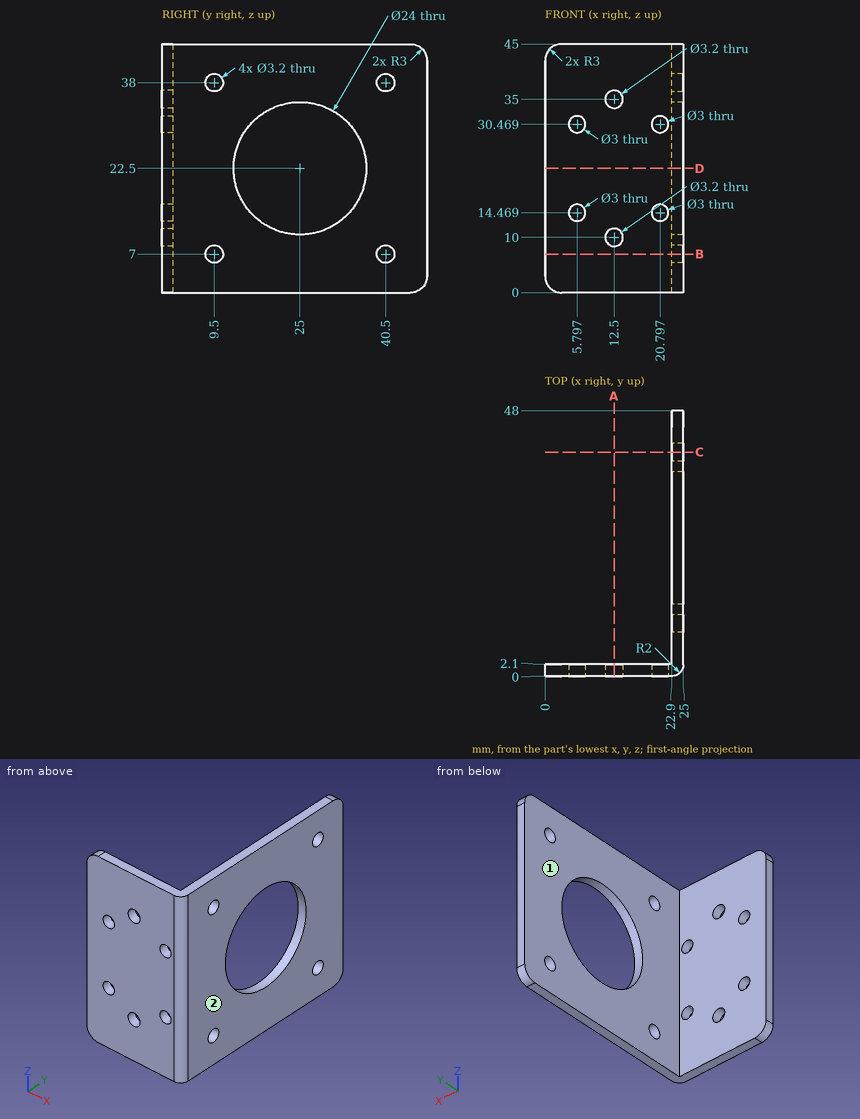
Part print with two shaded views. Sizes in mm from the minimum x, y, z corner. A direction names the side the tool comes from. Coordinates: 2 decimals unless noted, no trailing zeros. Write each loop counter-clockwise with the first axis right and the second up, starting at its lowest first coordinate (ties: lowest second). Pieces come first, ordered by that corner, then holes. Notation, with made-up numbers: M 34.5,28.25 L 45.5,28.25 A35 ccw 45.5,60.25 Z; hole C 66,-10 d5. An arc over 180 degrees is marked long. Return JSON: item names as keys, results as strings.
Item 1: Which spindle directions (+Z, -Z, +X, -X, +Y, -Y) get a long thin tool onto all of the face, cutting with end or side? Do the marked faces 1 and 2. Say none if no direction does.
Findings below:
{"face 1": "+Z, -Z, -X, +Y", "face 2": "+Z, -Z, +X, +Y, -Y"}
Item 2: Slice it at C-C, the plane y = 40.5. Write the cut outline in (x, z).
Findings below:
{"outline": "M 22.9,0 L 25,0 L 25,5.4 L 22.9,5.4 Z; M 22.9,8.6 L 25,8.6 L 25,36.4 L 22.9,36.4 Z; M 22.9,39.6 L 25,39.6 L 25,45 L 22.9,45 Z"}
Item 3: Slice it at D-D, the plane z = 22.5. Write the cut outline in (x, y).
Findings below:
{"outline": "M 0,0 L 23,0 A2 ccw 25,2 L 25,13 L 22.9,13 L 22.9,2.1 L 0,2.1 Z; M 22.9,37 L 25,37 L 25,48 L 22.9,48 Z"}
Item 4: Probe line 1 (Y direction, x = 12.5, z = 39); line 2 (X direction, y = 6, z = 30); line 3 (Y direction, x = 24.5, z = 22.5). List the from-to ranges inside material, lowest first. Write a range as from..to.
Findings below:
{"line 1": "y = 0..2.1", "line 2": "x = 22.9..25", "line 3": "y = 0.68..13, 37..48"}
Item 5: Slice it at B-B, the plane z = 7. Write the cut outline in (x, y), and give its area (3 significant figures).
Findings below:
{"outline": "M 0,0 L 23,0 A2 ccw 25,2 L 25,7.9 L 22.9,7.9 L 22.9,2.1 L 0,2.1 Z; M 22.9,11.1 L 25,11.1 L 25,38.9 L 22.9,38.9 Z; M 22.9,42.1 L 25,42.1 L 25,48 L 22.9,48 Z", "area": "135 mm2"}
Item 6: Slice it at A-A, the plane x = 12.5. Write the cut outline in (y, z).
Findings below:
{"outline": "M 0,0 L 2.1,0 L 2.1,8.4 L 0,8.4 Z; M 0,11.6 L 2.1,11.6 L 2.1,33.4 L 0,33.4 Z; M 0,36.6 L 2.1,36.6 L 2.1,45 L 0,45 Z"}
Item 7: Drop flat-ended pins along their axis: pin 1 Ø2.5 at (x, z) = (5.8, 30.47) entering from +Y; pin 2 Ø2 at (y, z) = (42, 36) entering from -X; pin 3 Ø3.5 at (x, z) = (5.8, 14.47) entering from +Y. Give the stop position or say it passes through.
Findings below:
{"pin 1": "passes through", "pin 2": "stops at x = 22.9", "pin 3": "stops at y = 2.1"}
